Read the model definition and answer for the solid it produces. Units are mm, in the model's axes. Round coordinates to 2 decimals unless told otherwise and drop trailing zeros. Order: outer loops, then holes, each group sorted by start corner. A loop starts at its lowest first (then second) coordinate and runs counter-clockwise, first axis right, second up. Notation, with made-up numbers: (-38, 77) -> (-5, 77) arc R21 ccw to (-5, 110) -> close; hole circle Ø10 at (-30.5, 46.25). An arc over 180 degrees is marked (long way). Use a Markdown table: item, result. Add a question column.
1. Given pin 1 (4 mm diameter, centred on x = -35.75, y = -35.75, fed in from -Z), flat-ended and moving along its own axis, determine where the tip first touches the part or whether it passes through.
2. Section A-A, the plane z = 6 is taken. Give the vertices of the cut face in (x, y), then the cut area to 3 significant figures.
3. Section B-B, the plane y = 23.5 is taken. Give the vertices of the cut face in (x, z).
4. Section C-C, the plane x = 32 is taken. Give the vertices of the cut face in (y, z).
5. Consider L1, parallel to Y at x = -0.5, z = 3; L2, parallel to Y at x = 32, z = 2.75; L3, parallel to X at y = -9.5, z = 6. Determine where each line is inside the solid, lowest interval first. Write a range as [from, to].
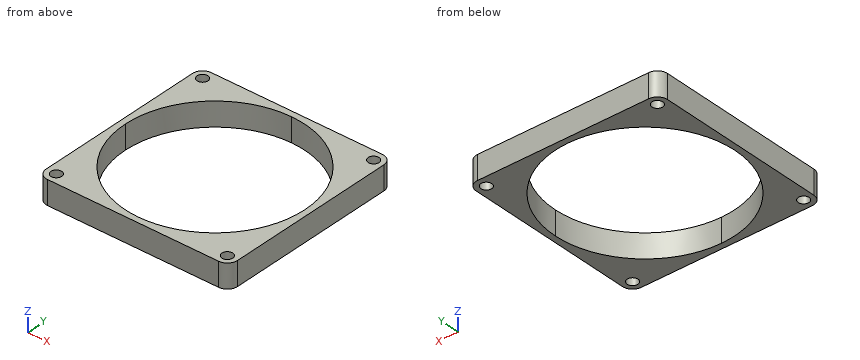
```python
from build123d import *

# Parameters (mm, degrees)
F0_R     = 2.25
F1_DEPTH = 10


with BuildPart() as f1:
    # F0 (on Top) → F1 (new body)
    with BuildSketch(Plane.XY):
        with BuildLine():
            ThreePointArc((0, 37.5), (26.516504, 26.516504), (37.5, 0))
            Line((37.5, 0), (40, 0))
            Line((40, 0), (40, 35.75))
            ThreePointArc((40, 35.75), (38.755204, 38.755204), (35.75, 40))
            Line((35.75, 40), (0, 40))
            Line((0, 40), (0, 37.5))
        make_face()
        with Locations((35.75, 35.75)):
            Circle(F0_R, mode=Mode.SUBTRACT)
    extrude(amount=F1_DEPTH)

    # F2: F1 across face


with BuildPart() as f1_1:
    add(f1.part)
    add(f1.part.mirror(Plane(origin=(38.75, 0, 5), x_dir=(1, 0, 0), z_dir=(0, -1, 0))))

    # F3: F1 across face


with BuildPart() as f1_2:
    add(f1_1.part)
    add(f1_1.part.mirror(Plane(origin=(0, 38.75, 5), x_dir=(0, -1, 0), z_dir=(-1, 0, 0))))


solid = f1_2.part
```
Verdict:
| question | item | result |
|---|---|---|
| 1 | pin 1 | passes through |
| 2 | outline | (-40, -35.75) arc R4.25 ccw to (-35.75, -40) -> (35.75, -40) arc R4.25 ccw to (40, -35.75) -> (40, 35.75) arc R4.25 ccw to (35.75, 40) -> (-35.75, 40) arc R4.25 ccw to (-40, 35.75) -> close; hole circle Ø4.5 at (-35.75, -35.75); hole circle Ø4.5 at (-35.75, 35.75); hole (-37.5, 0) arc R37.5 ccw to (0, -37.5) arc R37.5 ccw to (37.5, 0) arc R37.5 ccw to (0, 37.5) arc R37.5 ccw to start; hole circle Ø4.5 at (35.75, -35.75); hole circle Ø4.5 at (35.75, 35.75) |
| 2 | area | 1,900 mm2 |
| 3 | outline | (-40, 0) -> (-29.22, 0) -> (-29.22, 10) -> (-40, 10) -> close; (29.22, 0) -> (40, 0) -> (40, 10) -> (29.22, 10) -> close |
| 4 | outline | (-40, 0) -> (-19.55, 0) -> (-19.55, 10) -> (-40, 10) -> close; (19.55, 0) -> (40, 0) -> (40, 10) -> (19.55, 10) -> close |
| 5 | L1 | y = [-40, -37.5], [37.5, 40] |
| 5 | L2 | y = [-40, -19.55], [19.55, 40] |
| 5 | L3 | x = [-40, -36.28], [36.28, 40] |
